Here's how the part is built. I have some questions about the finished solid (model axes, mm). A direction names the side the tool comes from. Coordinates: 2 decimals unless noted, no trailing zeros. Write each loop counter-clockwise with the first axis right and the second up, starting at its lowest first coordinate (ties: lowest second). Pieces come first, ordered by that corner, then holes. Notation, with made-up numbers: (-7, 70) -> (44, 70) arc R19 ccw to (44, 102) -> close; hole circle Ø11 at (-16, 42). An arc over 180 degrees is marked (long way). Answer in a Markdown table with one row per item. Add a question column.
Autodesk Inventor part; units mm, degrees
ref_plane "YZ Plane" through (0, 0, 0) normal (1, 0, 0) x (0, 1, 0)
ref_plane "XZ Plane" through (0, 0, 0) normal (0, 1, 0) x (-1, 0, 0)
ref_plane "XY Plane" through (0, 0, 0) normal (0, 0, 1) x (1, 0, 0)
sketch "Sketch1" plane through (0, 0, 0) normal (0, 1, 0) x (-1, 0, 0)
  line L0 (58.5724, -67.15) -> (66.5724, -67.15)
  line L1 (58.5724, 20.85) -> (58.5724, -67.15)
  line L2 (66.5724, 20.85) -> (58.5724, 20.85)
  line L3 (66.5724, 20.85) -> (66.5724, -67.15)
  line L4 (-7.3261, 20.85) -> (0.6739, 20.85)
  line L5 (-7.3261, -67.15) -> (-7.3261, 20.85)
  line L6 (0.6739, -67.15) -> (-7.3261, -67.15)
  line L7 (0.6739, 20.85) -> (0.6739, -67.15)
  line L8 (58.5724, 20.85) -> (0.6739, 20.85)
  line L9 (58.5724, -67.15) -> (0.6739, -67.15)
  point P0 (0, 0)
extrude "Extrusion1" add sketch "Sketch1" against normal blind 5
sketch "Sketch2" plane through (0, -5, 0) normal (0, -1, 0) x (1, 0, 0)
  line L0 (-58.5724, 20.85) -> (-58.5724, -67.15)
  line L1 (-0.6739, -67.15) -> (-0.6739, 20.85)
  line L2 (-79.1232, -42.15) -> (-79.1232, -48.15)
  line L3 (-79.1232, 1.85) -> (-79.1232, -4.15)
  line L4 (-79.1232, 1.85) -> (-0.6739, 1.85)
  line L5 (-0.6739, 1.85) -> (-0.6739, -4.15)
  line L6 (-0.6739, -4.15) -> (-79.1232, -4.15)
  line L7 (-79.1232, -4.15) -> (-79.1232, 1.85)
  line L8 (-79.1232, -42.15) -> (-0.6739, -42.15)
  line L9 (-0.6739, -42.15) -> (-0.6739, -48.15)
  line L10 (-0.6739, -48.15) -> (-79.1232, -48.15)
  line L11 (-79.1232, -48.15) -> (-79.1232, -42.15)
  line L12 (-58.5724, 1.85) -> (-58.5724, -4.15)
  line L13 (-58.5724, -42.15) -> (-58.5724, -48.15)
  point P0 (0, 0)
  point P1 (-0.6739, -2.6877)
  point P2 (-58.5724, -2.6877)
  point P3 (-0.6739, -8.6877)
  point P4 (-58.5724, -8.6877)
extrude "Extrusion2" cut sketch "Sketch2" against normal blind 5 contours L4 L1 L6 L0 | L8 L1 L10 L0
fillet "Fillet1" radius 2 8 edges at (-58.5724, -2.5, 1.85) (-58.5724, -2.5, -4.15) (-0.6739, -2.5, 1.85) (-0.6739, -2.5, -4.15) (-0.6739, -2.5, -42.15) (-0.6739, -2.5, -48.15) (-58.5724, -2.5, -42.15) (-58.5724, -2.5, -48.15)
sketch "Sketch3" plane through (0, -5, 0) normal (0, -1, 0) x (1, 0, 0)
  circle A0 centre (-8.8162, 11.0267) radius 6
  circle A1 centre (-53.0208, 11.0267) radius 6
  circle A2 centre (-53.0208, -54.8709) radius 6
  circle A3 centre (-7.7929, -54.8709) radius 6
  point P0 (0, 0)
extrude "Extrusion3" cut sketch "Sketch3" against normal blind 10
properties part number "КВ33.000.105 - Заслонка"
Q1. I'm going to push flat-ended pins straight in: P1, Ø14, axis at x = -53.02, z = -54.87, coming from the +Y side; P2, Ø7, axis at x = -7.79, z = -54.87, coming from the +Y side. Where does each tip first touch, or does it pass through?
Q2. Imagine slicing it at A-A on x = -32. Please give me the cut outline in (y, z), plus the area to 3 significant figures.
Q3. If we mould it in two halves opening along Z, with no side actions, what happens to faces 1 (the flat face through (7.326, -2, -24)), 2 (the flat face through (-29, -2, -67.15)), 3 (the flat face through (-29, -3, -4.15))? For each: pulls with the +Z half, pulls with the -Z half, needs draft (parallel to the pull), parting line crosses it, or undercut.
Q4. Imagine slicing it at D-D on y = -1.2. Please give me the cut outline in (x, z), plus the area to 3 significant figures.
Q5. Imagine slicing it at C-C on x = -51. Please give me the cut outline in (y, z), plus the area to 3 significant figures.
Q6. For faces 4 (the flat face through (-29, -5, -23)), 5 (the cylindrical face through (-58, -2.46, 1.25)), which set-ups out of +Z, -Z, +X, -X, +Y, -Y let a thin tool reach every point of the face, with its end or its side?
Q7. Imagine slicing it at B-B on z = -59.5. Please give me the cut outline in (x, y).
Q8. I need wall thicknesses on line 1 (Z direction, x = -23.5, y = -0.2); line 2 (X direction, y = -2, z = -55); line 3 (X direction, y = -4.3, z = -46). Which ranges of each line are inside material? Lowest first, please. Write a range as [from, to].
Result sheet:
| question | item | result |
|---|---|---|
| 1 | P1 | stops at y = 0 |
| 1 | P2 | passes through |
| 2 | outline | (-5, -67.15) -> (0, -67.15) -> (0, -48.15) -> (-5, -48.15) -> close; (-5, -42.15) -> (0, -42.15) -> (0, -4.15) -> (-5, -4.15) -> close; (-5, 1.85) -> (0, 1.85) -> (0, 20.85) -> (-5, 20.85) -> close |
| 2 | area | 380 mm^2 |
| 3 | face 1 | needs draft |
| 3 | face 2 | pulls with the -Z half |
| 3 | face 3 | undercut |
| 4 | outline | (-66.57, -67.15) -> (7.33, -67.15) -> (7.33, 20.85) -> (-66.57, 20.85) -> close; hole circle Ø12 at (-53.02, -54.87); hole circle Ø12 at (-53.02, 11.03); hole (-58.57, -46.15) arc R2 ccw to (-56.57, -48.15) -> (-2.67, -48.15) arc R2 ccw to (-0.67, -46.15) -> (-0.67, -44.15) arc R2 ccw to (-2.67, -42.15) -> (-56.57, -42.15) arc R2 ccw to (-58.57, -44.15) -> close; hole (-58.57, -2.15) arc R2 ccw to (-56.57, -4.15) -> (-2.67, -4.15) arc R2 ccw to (-0.67, -2.15) -> (-0.67, -0.15) arc R2 ccw to (-2.67, 1.85) -> (-56.57, 1.85) arc R2 ccw to (-58.57, -0.15) -> close; hole circle Ø12 at (-8.82, 11.03); hole circle Ø12 at (-7.79, -54.87) |
| 4 | area | 5,360 mm^2 |
| 5 | outline | (-5, -67.15) -> (0, -67.15) -> (0, -60.52) -> (-5, -60.52) -> close; (-5, -49.22) -> (0, -49.22) -> (0, -48.15) -> (-5, -48.15) -> close; (-5, -42.15) -> (0, -42.15) -> (0, -4.15) -> (-5, -4.15) -> close; (-5, 1.85) -> (0, 1.85) -> (0, 5.38) -> (-5, 5.38) -> close; (-5, 16.68) -> (0, 16.68) -> (0, 20.85) -> (-5, 20.85) -> close |
| 5 | area | 267 mm^2 |
| 6 | face 4 | +Z, -Z, +X, -X, -Y |
| 6 | face 5 | +Y, -Y |
| 7 | outline | (-66.57, -5) -> (-56.84, -5) -> (-56.84, 0) -> (-66.57, 0) -> close; (-49.2, -5) -> (-11.61, -5) -> (-11.61, 0) -> (-49.2, 0) -> close; (-3.98, -5) -> (7.33, -5) -> (7.33, 0) -> (-3.98, 0) -> close |
| 8 | line 1 | z = [-67.15, -48.15], [-42.15, -4.15], [1.85, 20.85] |
| 8 | line 2 | x = [-66.57, -59.02], [-47.02, -13.79], [-1.79, 7.33] |
| 8 | line 3 | x = [-66.57, -58.57], [-0.67, 7.33] |
